from build123d import *

# Parameters (mm, degrees)
F0_R     = 74.1
F0_R_2   = 71.09
F1_DEPTH = 260
F2_R     = 78.65
F2_R_2   = 73.4
F3_DEPTH = 27
F4_R     = 74.1
F4_R_2   = 73.4
F5_DEPTH = 27
F6_SIZE  = 2
F7_R     = 95.050876
F7_R_2   = 7.411158
F8_DEPTH = 80


with BuildPart() as f1:
    # F0 (on Front) → F1 (new body)
    with BuildSketch(Plane.XZ):
        Circle(F0_R)
        Circle(F0_R_2, mode=Mode.SUBTRACT)
    extrude(amount=F1_DEPTH)

    # F2 (on Front) → F3 (cut)
    with BuildSketch(Plane.XZ):
        Circle(F2_R)
        Circle(F2_R_2, mode=Mode.SUBTRACT)
    extrude(amount=F3_DEPTH, mode=Mode.SUBTRACT)

    # F4 (on face) → F5 (cut)
    with BuildSketch(Plane.XZ.offset(260)):
        Circle(F4_R)
        Circle(F4_R_2, mode=Mode.SUBTRACT)
    extrude(amount=-F5_DEPTH, mode=Mode.SUBTRACT)

    # F6
    f6_edges = [f1.edges().sort_by_distance(p)[0] for p in [
        (-71.09, -260, 0),
        (-71.09, 0, 0),
    ]]
    chamfer(f6_edges, length=F6_SIZE)

    # F7 (on face) → F8 (cut)
    with BuildSketch(Plane.XZ.offset(260)):
        Circle(F7_R)
        Circle(F7_R_2, mode=Mode.SUBTRACT)
    extrude(amount=-F8_DEPTH, mode=Mode.SUBTRACT)


solid = f1.part
Design review of the part built by this model. Coordinates are the model's own, in mm. A direction names the side the tool comes from. Coordinates: 2 decimals unless noted, no trailing zeros. Loops run counter-clockwise (first coordinate to the right, second up) from the corner with the lowest first, then second, coordinate; pieces in that order, holes last. Notation, with made-up numbers: M -39.5,-34 L 8.5,-34 A19 ccw 8.5,-21 Z; hole C 69.25,32 d3. An arc over 180 degrees is marked long. Answer as CSV lines item,"result".
Item 1: For P1, Ø12, axis at x = -38, y = -59, coming from the +Z side; P2, Ø5, axis at x = 9.5, y = -57.5, coming from the +Z side; P3, Ø10, axis at y = -152, z = -28.5, coming from the +X side, all flat-tipped, find the tip position at first contact; note any pin that passes through.
Answer list:
P1,"z = 66.83"
P2,"z = 73.77"
P3,"x = 70.27"
Item 2: Add section D-D on y = -136. State the section outline as (x, z) points.
Answer list:
outline,"C 0,0 d148.2; hole C 0,0 d142.18"
Item 3: Add section B-B on x = 0. State the section outline as (y, z) points, plus the area to 3 significant figures.
Answer list:
outline,"M -180,-74.1 L -27,-74.1 L -27,-73.4 L 0,-73.4 L 0,-73.09 L -2,-71.09 L -180,-71.09 Z; M -180,71.09 L -2,71.09 L 0,73.09 L 0,73.4 L -27,73.4 L -27,74.1 L -180,74.1 Z"
area,"1,040 mm²"
Item 4: Machinability: for faces 1 (the face through (-28, -180, 66)), 2 (the face through (70.01, -13.31, 22.05)), which of the approach directions +Z, -Z, +X, -X, +Y, -Y give a long, thin tool a straight path to every point of the face, cutting with its end or side? Answer none if there is none.
Answer list:
face 1,"+Z, -Z, +X, -X, -Y"
face 2,"+Y"
Item 5: Add section C-C on y = -24. State the section outline as (x, z) points, plus the area to 3 significant figures.
Answer list:
outline,"C 0,0 d146.8; hole C 0,0 d142.18"
area,"1,050 mm²"
Item 6: The part is to be moulded in two halves that separate along Z. For faces 3 (the face through (68.45, -102.43, -28.38)), 4 (the face through (-71.7, -27, 16.8)), 5 (the face through (67.81, -89.75, 21.35)), say which applies: pulls with the +Z half, pulls with the -Z half, needs draft (parallel to the pull), parting line crosses it, or undercut.
Answer list:
face 3,"parting line crosses it"
face 4,"needs draft"
face 5,"undercut"
Item 7: For probe 1 along X at (y, z) = (-122, -0.5); probe 2 along X at (y, z) = (-130.5, 2.5), list the stretches that pass through material, from the lowest coordinate up.
Answer list:
probe 1,"-74.1 to -71.09, 71.09 to 74.1"
probe 2,"-74.06 to -71.05, 71.05 to 74.06"
Item 8: Add section A-A on z = 0. State the section outline as (x, y) points, plus the area to 3 significant figures.
Answer list:
outline,"M -74.1,-180 L -71.09,-180 L -71.09,-2 L -73.09,0 L -73.4,0 L -73.4,-27 L -74.1,-27 Z; M 71.09,-180 L 74.1,-180 L 74.1,-27 L 73.4,-27 L 73.4,0 L 73.09,0 L 71.09,-2 Z"
area,"1,040 mm²"
